CAD build for the part. Positions are in the model's coordinates, mm. A direction names the side the tool comes from. Give positions to 0.01 mm unless a question says otherwise; leave off trailing zeros. Order: outer loops, then holes, each group sorted by start corner. A loop starts at its lowest first (then second) coordinate and runs counter-clockwise, first axis right, second up.
```python
from build123d import *

# Parameters (mm, degrees)
SALIENTE_EXTRUIR1_DEPTH = 50
VACIADO2_T              = -2
CHAFL_N3_SIZE           = 1.5
CROQUIS2_R              = 7.5
SALIENTE_EXTRUIR2_DEPTH = 6
CROQUIS4_R              = 5
CORTAR_EXTRUIR2_DEPTH   = 5
REDONDEO1_R             = 0.5
CROQUIS5_R              = 3
CORTAR_EXTRUIR3_DEPTH   = 10
CROQUIS6_W              = 6
CROQUIS6_H              = 6
CORTAR_EXTRUIR4_DEPTH   = 10
CROQUIS7_W              = 4
CROQUIS7_H              = 4
SALIENTE_EXTRUIR3_DEPTH = 1


with BuildPart() as part:
    # Croquis1 → Saliente-Extruir1 (new body)
    with BuildSketch(Plane(origin=(0, 0, 0), x_dir=(1, 0, 0), z_dir=(0, 1, 0))):
        Polygon((-25, -32.5), (25, -32.5), (32.5, -25), (32.5, 25), (25, 32.5), (-25, 32.5), (-32.5, 25), (-32.5, -25), align=None)
    extrude(amount=SALIENTE_EXTRUIR1_DEPTH)

    # Vaciado2
    vaciado2_openings = [part.faces().sort_by_distance(p)[0] for p in [
        (0, 0, 0),
    ]]
    offset(amount=VACIADO2_T, openings=vaciado2_openings, kind=Kind.INTERSECTION)

    # Chaflán3
    chafl_n3_edges = [part.edges().sort_by_distance(p)[0] for p in [
        (-28.75, 50, -28.75),
        (-32.5, 50, 0),
        (-28.75, 50, 28.75),
        (0, 50, 32.5),
        (28.75, 50, 28.75),
        (32.5, 50, 0),
        (28.75, 50, -28.75),
        (0, 50, -32.5),
    ]]
    chamfer(chafl_n3_edges, length=CHAFL_N3_SIZE)

    # Croquis2 → Saliente-Extruir2 (add)
    with BuildSketch(Plane.XY.offset(32.5)):
        with Locations(Location((13, 35, 0), (0, 0, 180))):
            Circle(CROQUIS2_R)
        with Locations(Location((-13, 35, 0), (0, 0, 180))):
            Circle(CROQUIS2_R)
    extrude(amount=SALIENTE_EXTRUIR2_DEPTH)

    # Croquis4 → Cortar-Extruir2 (cut)
    with BuildSketch(Plane(origin=(0, 0, 30.5), x_dir=(-1, 0, 0), z_dir=(0, 0, -1))):
        with Locations((-13, 35)):
            Circle(CROQUIS4_R)
        with Locations(Location((13, 35, 0), (0, 0, 180))):
            Circle(CROQUIS4_R)
    extrude(amount=-CORTAR_EXTRUIR2_DEPTH, mode=Mode.SUBTRACT)

    # Redondeo1
    redondeo1_edges = [part.edges().sort_by_distance(p)[0] for p in [
        (20.5, 35, 38.5),
        (-5.5, 35, 38.5),
    ]]
    fillet(redondeo1_edges, radius=REDONDEO1_R)

    # Croquis5 → Cortar-Extruir3 (cut)
    with BuildSketch(Plane.XY.offset(32.5)):
        with Locations((0, 17.9)):
            Circle(CROQUIS5_R)
    extrude(amount=-CORTAR_EXTRUIR3_DEPTH, mode=Mode.SUBTRACT)

    # Croquis6 → Cortar-Extruir4 (cut)
    with BuildSketch(Plane(origin=(0, 0, -32.5), x_dir=(-1, 0, 0), z_dir=(0, 0, -1))):
        with Locations((-18, 6)):
            Rectangle(CROQUIS6_W, CROQUIS6_H)
    extrude(amount=-CORTAR_EXTRUIR4_DEPTH, mode=Mode.SUBTRACT)

    # Croquis7 → Saliente-Extruir3 (add)
    with BuildSketch(Plane(origin=(0, 0, 30.5), x_dir=(-1, 0, 0), z_dir=(0, 0, -1))):
        with Locations((-11.58, 9.3)):
            Rectangle(CROQUIS7_W, CROQUIS7_H)
        with Locations((-11.58, 26.8)):
            Rectangle(CROQUIS7_W, CROQUIS7_H)
        with Locations((11.43, 9.3)):
            Rectangle(CROQUIS7_W, CROQUIS7_H)
        with Locations((11.43, 26.8)):
            Rectangle(CROQUIS7_W, CROQUIS7_H)
    extrude(amount=SALIENTE_EXTRUIR3_DEPTH)


solid = part.part
```
Item 1: Tool access for faces 4 (the face through (-8.381, 36.915, 32.965)), 5 (the face through (14.63, 42.32, 35.21)), 6 (the face through (18, 3, -32)), 7 (the face through (12, 27, 29.5)): list every direction of +Z, -Z, +X, -X, +Y, -Y with a clear straight run to the whole face (end or side of a thin tool).
Item 2: Slice it at C-C (y = 45.5). Give the cut face in (x, z).
Item 3: Slice it at A-A (y = 17.9). Give the cut face in (x, z), and give its area (3 significant figures).
Item 4: Drop flat-ended pins along their axis: pin 1 Ø0.8 at (y, z) = (10, 30) entering from +X; pin 2 Ø1.1 at (y, z) = (27.5, 30) entering from -X; pin 3 Ø0.5 at (x, z) = (11, 30) entering from -Y; pin 4 Ø2 at (x, z) = (19, -31.5) entering from +Y. Give the stop position or say it passes through.
Item 5: Slice it at D-D (z = -13.5). Give the cut face in (x, y).
Item 6: Slice it at B-B (x = 0). Give the cut face in (y, z).
Item 7: Two-plate mould, pull along X, no slides. Class faces 1 (the face through (-13, 35, 38.5)), 2 (the face through (13, 35, 35.5)), 3 (the face through (-32.5, 24, 0)): released by +X, released by -X, zero draft, split by the parting line, or undercut.
Item 8: Wall check: L1, parallel to X at y = 15, z = -15.5; L2, parallel to Y at x = -13, z = 33.95. Give the ranges that are in metal, low to high.
A:
1. face 4: none
1. face 5: +Z
1. face 6: -Z
1. face 7: -Y
2. outline: (-32.5, -25) - (-25, -32.5) - (25, -32.5) - (32.5, -25) - (32.5, 25) - (25, 32.5) - (-25, 32.5) - (-32.5, 25) - close; hole (-30.5, -24.17) - (-24.17, -30.5) - (24.17, -30.5) - (30.5, -24.17) - (30.5, 24.17) - (24.17, 30.5) - (-24.17, 30.5) - (-30.5, 24.17) - close
3. outline: (-32.5, -25) - (-25, -32.5) - (25, -32.5) - (32.5, -25) - (32.5, 25) - (25, 32.5) - (3, 32.5) - (3, 30.5) - (24.17, 30.5) - (30.5, 24.17) - (30.5, -24.17) - (24.17, -30.5) - (-24.17, -30.5) - (-30.5, -24.17) - (-30.5, 24.17) - (-24.17, 30.5) - (-3, 30.5) - (-3, 32.5) - (-25, 32.5) - (-32.5, 25) - close
3. area: 460 mm2
4. pin 1: stops at x = 27.9
4. pin 2: stops at x = -28.05
4. pin 3: stops at y = 7.3
4. pin 4: stops at y = 50
5. outline: (-32.5, 0) - (-30.5, 0) - (-30.5, 48) - (30.5, 48) - (30.5, 0) - (32.5, 0) - (32.5, 48.5) - (31, 50) - (-31, 50) - (-32.5, 48.5) - close
6. outline: (0, -32.5) - (48.5, -32.5) - (50, -31) - (50, 31) - (48.5, 32.5) - (20.9, 32.5) - (20.9, 30.5) - (48, 30.5) - (48, -30.5) - (0, -30.5) - close; (0, 30.5) - (14.9, 30.5) - (14.9, 32.5) - (0, 32.5) - close
7. face 1: zero draft
7. face 2: undercut
7. face 3: released by -X
8. L1: x = -32.5 to -30.5, 30.5 to 32.5
8. L2: y = 27.5 to 30, 40 to 42.5
